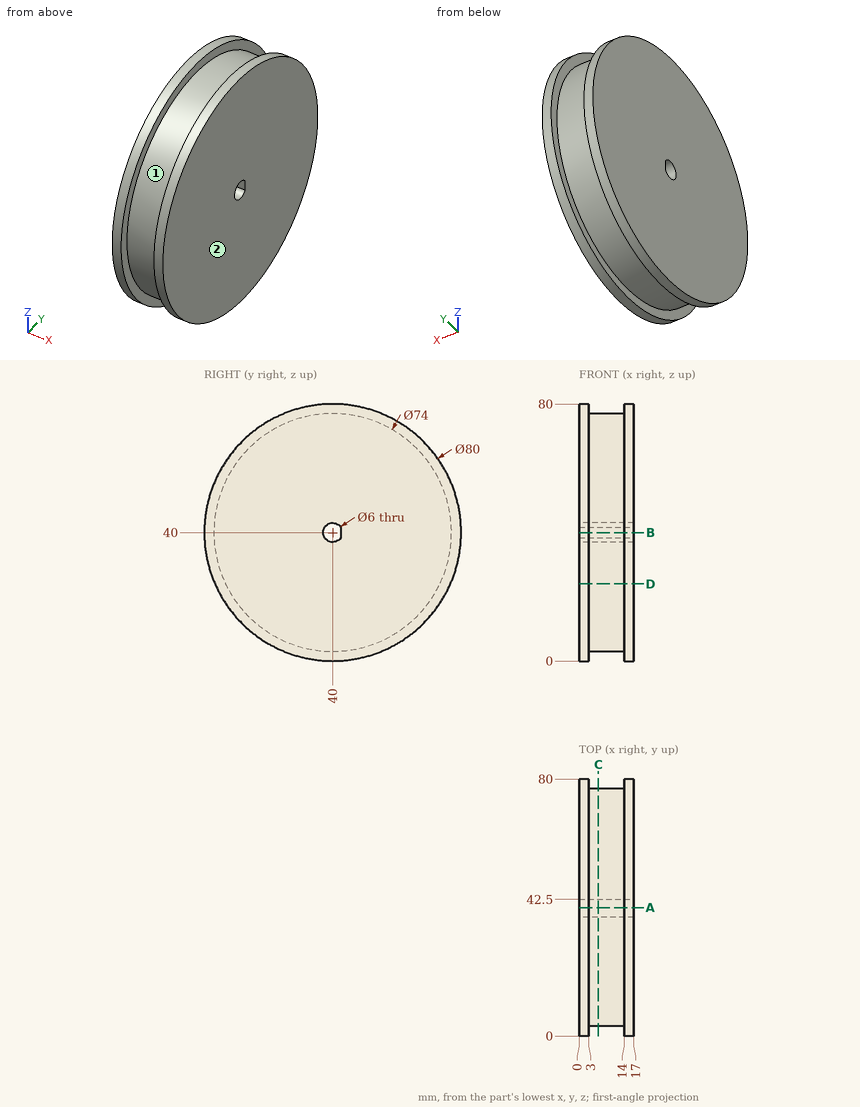
Geometry: see drawing. Coordinates: mm, zero at the bounding-box minimum. A direction names the side the tool comes from. Give positions to 0.01 mm unless a question says otherwise; leave off trailing zeros. Write each loop counter-clockwise with the first axis right and the second up, starting at its lowest first coordinate (ties: lowest second). Pieces come first, ordered by that corner, then holes. Notation, with made-up numbers: (8, 28.25) - (48, 28.25) arc R14 ccw to (48, 49.25) - close; hole circle Ø1 at (-23.75, -32). An arc over 180 degrees is marked (long way). Return JSON: item names as keys, results as strings. Group by question number.
1) Section A-A on y = 40. Return the cut outline in (x, z).
2) Section B-B on z = 40. Return the cut outline in (x, y), plus the area to 3 significant figures.
3) Section D-D on z = 24. Return the cut outline in (x, y), plus the area to 3 significant figures.
4) First-contact query: P1, Ø3.5, axis at x = 11.5, z = 39, coming from the -Y side; P2, Ø5, axis at x = 6, z = 34.5, coming from the +Y side; P3, Ø4, axis at x = 13, y = 18, coming from the -Z side. Flat tips, straight axial feed; report the tip coordinate or a pass-through.
5) Set-up query: the marked faces 1 and 2. Return all of +Z, -Z, +X, -X, +Y, -Y with unobstructed straight access to the full face (end or side cutting, diameter ignored); none if empty.
6) Section C-C on x = 6. Return the cut outline in (y, z), plus the area to 3 significant figures.
7) Line query: line 1 (Y direction, x = 9.25, z = 40); line 2 (Y direction, x = 16, z = 42.5); line 3 (Y direction, x = 10.5, z = 63.5). Output: solid intervals per line, ascending.
Filled in:
{
 "1": {"outline": "(0, 0) - (3, 0) - (3, 3) - (14, 3) - (14, 0) - (17, 0) - (17, 37) - (0, 37) - close; (0, 43) - (17, 43) - (17, 80) - (14, 80) - (14, 77) - (3, 77) - (3, 80) - (0, 80) - close"},
 "2": {"outline": "(0, 0) - (3, 0) - (3, 3) - (14, 3) - (14, 0) - (17, 0) - (17, 37) - (0, 37) - close; (0, 42.5) - (17, 42.5) - (17, 80) - (14, 80) - (14, 77) - (3, 77) - (3, 80) - (0, 80) - close", "area": "1,200 mm^2"},
 "3": {"outline": "(0, 3.34) - (3, 3.34) - (3, 6.64) - (14, 6.64) - (14, 3.34) - (17, 3.34) - (17, 76.66) - (14, 76.66) - (14, 73.36) - (3, 73.36) - (3, 76.66) - (0, 76.66) - close", "area": "1,170 mm^2"},
 "4": {"P1": "stops at y = 3", "P2": "stops at y = 76.88", "P3": "stops at z = 5.52"},
 "5": {"face 1": "none", "face 2": "+Z, -Z, +X, +Y, -Y"},
 "6": {"outline": "circle Ø74 at (40, 40); hole (42.5, 38.34) - (42.5, 41.66) arc R3 ccw (long way) to start", "area": "4,270 mm^2"},
 "7": {"line 1": "y = 3 to 37, 42.5 to 77", "line 2": "y = 0.08 to 38.34, 41.66 to 79.92", "line 3": "y = 11.42 to 68.58"}
}
